from build123d import *

# Parameters (mm, degrees)
SKETCH1_W                      = 22
SKETCH1_H                      = 40
SKETCH1_R                      = 1.5
BOSS_EXTRUDE1_DEPTH            = 5
BOSS_EXTRUDE3_DEPTH            = 40
FILLET1_R                      = 2
CUT_EXTRUDE1_REACH             = 34.746
SKETCH9_R                      = 1.5
CUT_EXTRUDE1_DIRECTION_2_REACH = 34.746


with BuildPart() as part:
    # Sketch1 → Boss-Extrude1 (new body)
    with BuildSketch(Plane(origin=(0, 0, 0), x_dir=(1, 0, 0), z_dir=(0, 1, 0))):
        Rectangle(SKETCH1_W, SKETCH1_H)
        with Locations(Location((0, 15, 0), (0, 0, 270))):
            Circle(SKETCH1_R, mode=Mode.SUBTRACT)
        with Locations(Location((0, -15, 0), (0, 0, 270))):
            Circle(SKETCH1_R, mode=Mode.SUBTRACT)
    extrude(amount=BOSS_EXTRUDE1_DEPTH)

    # Sketch4 → Boss-Extrude3 (add)
    with BuildSketch(Plane(origin=(0, 0, -20), x_dir=(-1, 0, 0), z_dir=(0, 0, -1))):
        Polygon((-11, 5), (-12, 5), (-12, 8.5), (-15, 8.5), (-15, 0), (-11, 0), align=None)
        Polygon((11, 0), (11, 5), (12, 5), (12, 8.5), (15, 8.5), (15, 0), align=None)
    extrude(amount=-BOSS_EXTRUDE3_DEPTH)

    # Fillet1
    fillet1_edges = [part.edges().sort_by_distance(p)[0] for p in [
        (15, 0, 0),
        (15, 8.5, 0),
        (-15, 0, 0),
        (-15, 8.5, 0),
    ]]
    fillet(fillet1_edges, radius=FILLET1_R)

    # Sketch6 → Loft1 section 0
    with BuildSketch(Plane(origin=(0, -20, 0), x_dir=(1, 0, 0), z_dir=(0, 1, 0))):
        with BuildLine():
            Line((11.018014761, 12.99270703), (-11, 7))
            Line((-11, 7), (-11, 3))
            Line((-11, 3), (11.018014761, 8.99270703))
            Line((11.018014761, 8.99270703), (11.018014761, 12.99270703))
        make_face()
    # Sketch2 → Loft1 section 1
    with BuildSketch(Plane.XZ):
        with BuildLine():
            Line((-11, 6), (11, 0.105117767))
            Line((11, 0.105117767), (11, -3.894882233))
            Line((11, -3.894882233), (-11, 2))
            Line((-11, 2), (-11, 6))
        make_face()
    loft()

    # Sketch9 → Cut-Extrude1 (cut, up to next)
    with BuildSketch(Plane(origin=(-0.191463171, 0.319826035, -0.703461542), x_dir=(-0.9706501889890885, -0.09953611163264846, 0.21893097792797594), z_dir=(-0.24049576007790016, 0.4017315961669107, -0.8836138942013866)), mode=Mode.PRIVATE) as cut_extrude1_sk1:
        with Locations(Location((-6.537902116, -11.132046288, 0), (0, 0, 90))):
            Circle(SKETCH9_R)
    cut_extrude1_tool1 = extrude(cut_extrude1_sk1.sketch, amount=-CUT_EXTRUDE1_REACH, mode=Mode.PRIVATE) & part.part
    # Sketch9 → Cut-Extrude1 (cut, up to next)
    with BuildSketch(Plane(origin=(-0.191463171, 0.319826035, -0.703461542), x_dir=(-0.9706501889890885, -0.09953611163264846, 0.21893097792797594), z_dir=(-0.24049576007790016, 0.4017315961669107, -0.8836138942013866)), mode=Mode.PRIVATE) as cut_extrude1_sk2:
        with Locations(Location((6.124840152, -9.767757873, 0), (0, 0, 90))):
            Circle(SKETCH9_R)
    cut_extrude1_tool2 = extrude(cut_extrude1_sk2.sketch, amount=-CUT_EXTRUDE1_REACH, mode=Mode.PRIVATE) & part.part
    add(cut_extrude1_tool1.solids().sort_by_distance((6.154553, -9.163274, -6.74213))[0], mode=Mode.SUBTRACT)
    add(cut_extrude1_tool2.solids().sort_by_distance((-6.13654, -9.181719, -3.405213))[0], mode=Mode.SUBTRACT)

    # Sketch9 → Cut-Extrude1 direction 2 (cut, up to next)
    with BuildSketch(Plane(origin=(-0.191463171, 0.319826035, -0.703461542), x_dir=(-0.9706501889890885, -0.09953611163264846, 0.21893097792797594), z_dir=(-0.24049576007790016, 0.4017315961669107, -0.8836138942013866)), mode=Mode.PRIVATE) as cut_extrude1_direction_2_sk1:
        with Locations(Location((-6.537902116, -11.132046288, 0), (0, 0, 90))):
            Circle(SKETCH9_R)
    cut_extrude1_direction_2_tool1 = extrude(cut_extrude1_direction_2_sk1.sketch, amount=CUT_EXTRUDE1_DIRECTION_2_REACH, mode=Mode.PRIVATE) & part.part
    # Sketch9 → Cut-Extrude1 direction 2 (cut, up to next)
    with BuildSketch(Plane(origin=(-0.191463171, 0.319826035, -0.703461542), x_dir=(-0.9706501889890885, -0.09953611163264846, 0.21893097792797594), z_dir=(-0.24049576007790016, 0.4017315961669107, -0.8836138942013866)), mode=Mode.PRIVATE) as cut_extrude1_direction_2_sk2:
        with Locations(Location((6.124840152, -9.767757873, 0), (0, 0, 90))):
            Circle(SKETCH9_R)
    cut_extrude1_direction_2_tool2 = extrude(cut_extrude1_direction_2_sk2.sketch, amount=CUT_EXTRUDE1_DIRECTION_2_REACH, mode=Mode.PRIVATE) & part.part
    add(cut_extrude1_direction_2_tool1.solids().sort_by_distance((6.154553, -9.163274, -6.74213))[0], mode=Mode.SUBTRACT)
    add(cut_extrude1_direction_2_tool2.solids().sort_by_distance((-6.13654, -9.181719, -3.405213))[0], mode=Mode.SUBTRACT)


solid = part.part
Geometry: final body of the model. Coordinates: model frame, mm. A direction names the side the tool comes from. Round coordinates to 2 decimals unless told otherwise and drop trailing zeros. Loops run counter-clockwise (first coordinate to the right, second up) from the corner with the lowest first, then second, coordinate; pieces in that order, holes last. Notation, with made-up numbers: (3.5, -30) - (18.5, -30) arc R13 ccw to (18.5, -7) - close; hole circle Ø8 at (13.5, 56). An arc over 180 degrees is marked (long way). Write each question's results on one line, items separated by ' | '. Start each with the question number.
1) Cut plane A-A on z = 15. Return loops of the section in (x, y).
2) Line query: probe 1 along X at (y, z) = (3.3, -15); probe 2 along Y at (x, z) = (4.5, 7); probe 3 along X at (y, z) = (1.55, 15). Output: solid intervals per line, ascending. Write a range as [from, to].
3) First-contact query: P1, Ø8, axis at x = -5.5, z = 3, coming from the -Y side; P2, Ø1.8, axis at x = 0, z = -15, coming from the +Y side; P3, Ø12, axis at x = 4, z = -8, coming from the +Y side; P4, Ø1.8, axis at y = 7.5, z = -5.5, coming from the -X side. Flat tips, straight axial feed; report the tip coordinate or a pass-through.
4) Cut plane C-C on z = -16. Return loops of the section in (x, y), then the cut area to 3 significant figures.
5) Mould query, pull axis X, two halves, no side actions, for faces 1 (the face through (0.07, 2.46, 13.5)), 2 (the face through (0, -20, -8)), 3 (the face through (15, 4, 0)), 4 (the face through (-15, 4, 0)). Classes: released by +X, released by -X, zero draft, split by the parting line, or undercut.
6) Cut plane B-B on y = 1.25. Return loops of the section in (x, z), then the cut area to 3 significant figures.
7) Cut plane D-D on x = 0. Count the separate pieces of the cut face and the enclosed holes in it, then the cut area to 3 significant figures.
8) Access query for faces 5 (the face through (14.4, 0.57, 0.28)), 6 (the face through (0, 5, 0)). Directions: +Z, -Z, +X, -X, +Y, -Y. A direction counts if a zero-diameter tool reaches every point of the face in a straight line with its end or side. Return the directions, or none.
Verdict:
1) outline: (-15, 2) arc R2 ccw to (-13, 0) - (-1.5, 0) - (-1.5, 5) - (-12, 5) - (-12, 8.5) - (-13, 8.5) arc R2 ccw to (-15, 6.5) - close; (1.5, 0) - (13, 0) arc R2 ccw to (15, 2) - (15, 6.5) arc R2 ccw to (13, 8.5) - (12, 8.5) - (12, 5) - (1.5, 5) - close
2) probe 1: x = [-15, -1.5], [1.5, 15] | probe 2: y = [0, 5] | probe 3: x = [-14.95, -1.5], [1.5, 14.95]
3) P1: stops at y = -12.57 | P2: passes through | P3: stops at y = 5 | P4: stops at x = -15
4) outline: (-15, 2) arc R2 ccw to (-13, 0) - (-1.12, 0) - (-1.12, 5) - (-12, 5) - (-12, 8.5) - (-13, 8.5) arc R2 ccw to (-15, 6.5) - close; (1.12, 0) - (13, 0) arc R2 ccw to (15, 2) - (15, 6.5) arc R2 ccw to (13, 8.5) - (12, 8.5) - (12, 5) - (1.12, 5) - close | area: 156 mm2
5) face 1: undercut | face 2: zero draft | face 3: released by +X | face 4: released by -X
6) outline: (-14.85, -20) - (14.85, -20) - (14.85, 20) - (-14.85, 20) - close; hole circle Ø3 at (0, -15); hole circle Ø3 at (0, 15) | area: 1,170 mm2
7) separate pieces: 3 | enclosed holes: 0 | area: 250 mm2
8) face 5: +Z, -Z, +X, -Y | face 6: +Z, -Z, +Y
